```python
from build123d import *
from build123d.topology import SkipClean

# Parameters (mm, degrees)
RESSALTO_EXTRUS_O4_DEPTH  = 8
ESBO_O7_W                 = 26
ESBO_O7_H                 = 8
RESSALTO_EXTRUS_O5_DEPTH  = 0.1
ESBO_O8_R                 = 5
CORTE_EXTRUS_O7_DEPTH     = 17.792855624
RESSALTO_EXTRUS_O6_DEPTH  = 7
ESBO_O10_R                = 1.5
CORTE_EXTRUS_O8_DEPTH     = 19.248287591
RESSALTO_EXTRUS_O7_DEPTH  = 1.5
ESBO_O12_W                = 2.553491136
ESBO_O12_H                = 15
RESSALTO_EXTRUS_O9_DEPTH  = 5.5
ESBO_O13_R                = 5
CORTE_EXTRUS_O9_DEPTH     = 22.04756518
ESBO_O14_R                = 1.468193857
ESBO_O14_R_2              = 1.484614178
RESSALTO_EXTRUS_O10_DEPTH = 4


with BuildPart() as part:
    # Esboço4 → Ressalto-extrusão4 (new body)
    with BuildSketch(Plane.XY):
        with BuildLine():
            Line((-13, -5), (13, -5))
            Line((13, -5), (13, -3))
            Line((13, -3), (6.32455532, -3))
            ThreePointArc((6.32455532, -3), (0, 7), (-6.32455532, -3))
            Line((-6.32455532, -3), (-13, -3))
            Line((-13, -3), (-13, -5))
        make_face()
    extrude(amount=RESSALTO_EXTRUS_O4_DEPTH)

    # Esboço7 → Ressalto-extrusão5 (add)
    with BuildSketch(Plane.XZ.offset(5)):
        with Locations((0, 4)):
            Rectangle(ESBO_O7_W, ESBO_O7_H)
    extrude(amount=RESSALTO_EXTRUS_O5_DEPTH)

    # Esboço8 → Corte-extrusão7 (cut, through all)
    with BuildSketch(Plane.XY.offset(8)):
        Circle(ESBO_O8_R)
    extrude(amount=-CORTE_EXTRUS_O7_DEPTH, mode=Mode.SUBTRACT)

    # Esboço9 → Ressalto-extrusão6 (add)
    with SkipClean():  # the faces are left unmerged after this step: merging them gives an invalid solid
        with BuildSketch(Plane(origin=(0, 0, 0), x_dir=(-1, 0, 0), z_dir=(0, 0, -1))):
            with BuildLine():
                Line((-6.32455532, -3), (-7.5, -3))
                Line((-7.5, -3), (-7.5, -5.1))
                Line((-7.5, -5.1), (0, -5.1))
                Line((0, -5.1), (7.5, -5.1))
                Line((7.5, -5.1), (7.5, -3))
                Line((7.5, -3), (6.32455532, -3))
                ThreePointArc((6.32455532, -3), (0, 7), (-6.32455532, -3))
            make_face()
            with BuildLine():
                ThreePointArc((5, 0), (4.74341649, -1.58113883), (4, -3))
                ThreePointArc((4, -3), (0, -5), (-4, -3))
                ThreePointArc((-4, -3), (-1.58113883, 4.74341649), (5, 0))
            make_face(mode=Mode.SUBTRACT)
        extrude(amount=RESSALTO_EXTRUS_O6_DEPTH)

    # Esboço10 → Corte-extrusão8 (cut, through all)
    with SkipClean():  # the faces are left unmerged after this step: merging them gives an invalid solid
        with BuildSketch(Plane(origin=(0, -3, 0), x_dir=(1, 0, 0), z_dir=(0, 1, 0))):
            with Locations(Location((-9, -4, 0), (0, 0, 180))):
                Circle(ESBO_O10_R)
            with Locations(Location((9, -4, 0), (0, 0, 180))):
                Circle(ESBO_O10_R)
        extrude(amount=-CORTE_EXTRUS_O8_DEPTH, mode=Mode.SUBTRACT)

    # Esboço11 → Ressalto-extrusão7 (add)
    # profile 1 of 3: a face of its own
    with SkipClean():  # the faces are left unmerged after this step: merging them gives an invalid solid
        with BuildSketch(Plane(origin=(0, 6.906344322, 0), x_dir=(0, 0, -1), z_dir=(0, 1, 0))):
            Polygon((7, 3), (7, 7), (-8, 7), (-8, -7), (7, -7), (7, -3), align=None)
        # profile 2 of 3: a face of its own
        with BuildSketch(Plane(origin=(0, 6.906344322, 0), x_dir=(0, 0, -1), z_dir=(0, 1, 0))):
            Polygon((7, 8), (7, 7), (7, 3), (11.5, 3), (11.5, 7), (11.5, 8), (9.25, 8), align=None)
            with BuildLine():
                ThreePointArc((10.25, 6), (8.542893219, 5.292893219), (9.25, 7))
                ThreePointArc((9.25, 7), (9.957106781, 6.707106781), (10.25, 6))
            make_face(mode=Mode.SUBTRACT)
        # profile 3 of 3: a face of its own
        with BuildSketch(Plane(origin=(0, 6.906344322, 0), x_dir=(0, 0, -1), z_dir=(0, 1, 0))):
            Polygon((11.5, -3), (7, -3), (7, -7), (7, -8), (9.25, -8), (11.5, -8), (11.5, -7), align=None)
            with BuildLine():
                ThreePointArc((10.25, -6), (9.957106781, -6.707106781), (9.25, -7))
                ThreePointArc((9.25, -7), (8.542893219, -5.292893219), (10.25, -6))
            make_face(mode=Mode.SUBTRACT)
        extrude(amount=-RESSALTO_EXTRUS_O7_DEPTH)

    # Esboço12 → Ressalto-extrusão9 (add)
    with SkipClean():  # the faces are left unmerged after this step: merging them gives an invalid solid
        with BuildSketch(Plane.XZ.offset(-5.406344322)):
            with Locations((-5.723254432, 0.5)):
                Rectangle(ESBO_O12_W, ESBO_O12_H)
            with Locations((5.723254432, 0.5)):
                Rectangle(ESBO_O12_W, ESBO_O12_H)
        extrude(amount=RESSALTO_EXTRUS_O9_DEPTH)

    # Esboço13 → Corte-extrusão9 (cut, through all)
    with SkipClean():  # the faces are left unmerged after this step: merging them gives an invalid solid
        with BuildSketch(Plane(origin=(0, 0, -7), x_dir=(-1, 0, 0), z_dir=(0, 0, -1))):
            with Locations(Location((0, 0, 0), (0, 0, 180))):
                Circle(ESBO_O13_R)
        extrude(amount=-CORTE_EXTRUS_O9_DEPTH, mode=Mode.SUBTRACT)

    # Esboço14 → Ressalto-extrusão10 (add)
    with SkipClean():  # the faces are left unmerged after this step: merging them gives an invalid solid
        with BuildSketch(Plane.XZ.offset(5.1)):
            Polygon((-13, 8), (-13, 0), (-7.5, 0), (-7.5, -7), (7.5, -7), (7.5, 0), (13, 0), (13, 8), align=None)
            with Locations((-9, 4)):
                Circle(ESBO_O14_R, mode=Mode.SUBTRACT)
            with Locations((9, 4)):
                Circle(ESBO_O14_R_2, mode=Mode.SUBTRACT)
        extrude(amount=RESSALTO_EXTRUS_O10_DEPTH)


solid = part.part
```
CAD build for the part. Positions are in the model's coordinates, mm. A direction names the side the tool comes from. Round coordinates to 2 decimals unless told otherwise and drop trailing zeros. Order: outer loops, then holes, each group sorted by start corner. A loop starts at its lowest first (then second) coordinate and runs counter-clockwise, first axis right, second up. Notation, with made-up numbers: (-36.75, 63.5) - (-3.75, 63.5) arc R15 cw to (-3.75, 78.5) - close; hole circle Ø8 at (85.5, 7.25). An arc over 180 degrees is marked (long way). Use CSV: the item, a comma, the result in double quotes. Start each with the question number.
1) Saw through at B-B (z = 4). Count the separate pieces of the cut face and the enclosed holes in it, and give its area (3 significant figures).
2) Saw through at A-A (x = 0). List the corners of the cut face in (y, z), and give its area (3 significant figures).
3) Pin check, flat tips, straight feed: pin 1 Ø2.5 at (y, z) = (1.5, 0) entering from -X; pin 2 Ø1.3 at (x, z) = (7, -4.5) entering from +Y; pin 3 Ø2 at (x, z) = (9.5, -1.5) entering from -Y; pin 4 Ø3 at (y, z) = (-7.5, -2.5) entering from -X. Stop position of each tip, or through.
4) Saw through at D-D (z = -7.5). List the corners of the cut face in (x, y), and give its area (3 significant figures).
5) Saw through at C-C (y = 3). List the corners of the cut face in (x, z).
6) Wall check: L1, parallel to X at y = 6.15, z = -9.25; L2, parallel to Z at x = -6, y = 6.15; L3, parallel to Y at x = 4, z = -3.75. Give the ranges that are in metal, low to high. Write a range as [from, to].
7) Tool access for faces 4 (the flat face through (3, 6, -9)), 5 (the flat face through (4.9, 5.406, -8.7)), 6 (the flat face through (-7.5, 6.2, -7)): list every direction of +Z, -Z, +X, -X, +Y, -Y with a clear straight run to the whole face (end or side of a thin tool).
8) Two-plate mould, pull along Z, no slides. Class faces 1 (the cylindrical face through (10.5, -4.04, 4.07)), 2 (the flat face through (-3, 6, -9)), 3 (the flat face through (6, 6, -11.5)): pulls with the +Z half, pulls with the -Z half, needs draft (parallel to the pull), parting line crosses it, or undercut.
Values follow:
1,separate pieces,"3"
1,enclosed holes,"1"
1,area,"181 mm2"
2,outline,"(-9.1, -7) - (-5, -7) - (-5, 8) - (-9.1, 8) - close; (5, -7) - (7, -7) - (7, 8) - (5, 8) - close"
2,area,"91.5 mm2"
3,pin 1,"stops at x = -7"
3,pin 2,"stops at y = 6.91"
3,pin 3,"passes through"
3,pin 4,"stops at x = -7.5"
4,outline,"(-8, 5.41) - (-3, 5.41) - (-3, 6.91) - (-8, 6.91) - close; (3, 5.41) - (8, 5.41) - (8, 6.91) - (3, 6.91) - close"
4,area,"15.0 mm2"
5,outline,"(-7, -7) - (-4, -7) - (-4, 8) - (-7, 8) - close; (4, -7) - (7, -7) - (7, 8) - (4, 8) - close"
6,L1,"x = [-8, -7], [-5, -3], [3, 5], [7, 8]"
6,L2,"z = [-11.5, -10.25], [-8.25, 8]"
6,L3,"y = [-9.1, -3], [3, 6.91]"
7,face 4,"-Z, +Y, -Y"
7,face 5,"-Z, +X, -X, -Y"
7,face 6,"+Z, -X, +Y"
8,face 1,"undercut"
8,face 2,"needs draft"
8,face 3,"pulls with the -Z half"
